from build123d import *

# Parameters (mm, degrees)
SKETCH1_W                                         = 133.096
SKETCH1_H                                         = 118.890132416
BOSS_EXTRUDE1_DEPTH                               = 10.16
SKETCH1_11_W                                      = 98.552
SKETCH1_11_H                                      = 57.404
SKETCH1_11_R                                      = 4.064
SKETCH1_11_W_2                                    = 18.542
SKETCH1_11_H_2                                    = 18.542
CUT_EXTRUDE1_DEPTH                                = 179.752998302
SKETCH1_12_R                                      = 13.75
SKETCH1_12_R_2                                    = 7.5
SKETCH1_12_R_3                                    = 4.064
CUT_EXTRUDE2_DEPTH                                = 1.7
CSK_FOR_M2_5_FLAT_HEAD_MACHINE_SCREW1_D           = 2.9
CSK_FOR_M2_5_FLAT_HEAD_MACHINE_SCREW1_DEPTH       = 5.08
CSK_FOR_M2_5_FLAT_HEAD_MACHINE_SCREW1_CSINK_D     = 5.5
CSK_FOR_M2_5_FLAT_HEAD_MACHINE_SCREW1_CSINK_ANGLE = 90
CSK_FOR_M2_5_FLAT_HEAD_MACHINE_SCREW1_TIP         = 0.871247898
SKETCH6_R                                         = 4.02
CUT_EXTRUDE3_DEPTH                                = 7.62


with BuildPart() as part:
    # Sketch1 → Boss-Extrude1 (new body)
    with BuildSketch(Plane.XY):
        with Locations((66.548, 59.445066208)):
            Rectangle(SKETCH1_W, SKETCH1_H)
    extrude(amount=-BOSS_EXTRUDE1_DEPTH)

    # Sketch1_11 → Cut-Extrude1 (cut, through all)
    with BuildSketch(Plane.XY):
        with Locations((78.74, 43.942)):
            Rectangle(SKETCH1_11_W, SKETCH1_11_H)
        with Locations((78.74, 98.4758)):
            Circle(SKETCH1_11_R)
        with Locations((16.289896793, 64.367970222)):
            Rectangle(SKETCH1_11_W_2, SKETCH1_11_H_2)
        with Locations((16.289896793, 42.362289183)):
            Rectangle(SKETCH1_11_W_2, SKETCH1_11_H_2)
        with BuildLine():
            Line((49.911, 74.803), (107.569, 74.803))
            ThreePointArc((107.569, 74.803), (110.744, 77.978), (107.569, 81.153))
            Line((107.569, 81.153), (49.911, 81.153))
            ThreePointArc((49.911, 81.153), (46.736, 77.978), (49.911, 74.803))
        make_face()
    extrude(amount=-CUT_EXTRUDE1_DEPTH, mode=Mode.SUBTRACT)

    # Sketch1_12 → Cut-Extrude2 (cut)
    # profile 1 of 3: a face of its own
    with BuildSketch(Plane.XY):
        with Locations((78.74, 98.4758)):
            Circle(SKETCH1_12_R)
        with Locations((78.74, 98.4758)):
            Circle(SKETCH1_12_R_2, mode=Mode.SUBTRACT)
    # profile 2 of 3: a face of its own
    with BuildSketch(Plane.XY):
        with Locations((78.74, 98.4758)):
            Circle(SKETCH1_12_R_2)
        with Locations((78.74, 98.4758)):
            Circle(SKETCH1_12_R_3, mode=Mode.SUBTRACT)
    # profile 3 of 3: a face of its own
    with BuildSketch(Plane.XY):
        with BuildLine():
            Line((49.911, 73.914), (107.569, 73.914))
            ThreePointArc((107.569, 73.914), (111.633, 77.978), (107.569, 82.042))
            Line((107.569, 82.042), (49.911, 82.042))
            ThreePointArc((49.911, 82.042), (45.847, 77.978), (49.911, 73.914))
        make_face()
        with BuildLine():
            ThreePointArc((107.569, 74.803), (110.744, 77.978), (107.569, 81.153))
            Line((107.569, 81.153), (49.911, 81.153))
            ThreePointArc((49.911, 81.153), (46.736, 77.978), (49.911, 74.803))
            Line((49.911, 74.803), (107.569, 74.803))
        make_face(mode=Mode.SUBTRACT)
    extrude(amount=-CUT_EXTRUDE2_DEPTH, mode=Mode.SUBTRACT)

    # CSK for M2.5 Flat Head Machine Screw1
    with Locations(Plane(origin=(0, 0, -10.16), x_dir=(-1, 0, 0), z_dir=(0, 0, -1))):
        with Locations((-109.250378399, 110.932782256), (-65.089376176, 110.932782256), (-6.474944958, 110.932782256), (-16.176873925, 29.217411756)):
            CounterSinkHole(CSK_FOR_M2_5_FLAT_HEAD_MACHINE_SCREW1_D / 2, CSK_FOR_M2_5_FLAT_HEAD_MACHINE_SCREW1_CSINK_D / 2, depth=CSK_FOR_M2_5_FLAT_HEAD_MACHINE_SCREW1_DEPTH, counter_sink_angle=CSK_FOR_M2_5_FLAT_HEAD_MACHINE_SCREW1_CSINK_ANGLE)
            with Locations((0, 0, -(CSK_FOR_M2_5_FLAT_HEAD_MACHINE_SCREW1_DEPTH + CSK_FOR_M2_5_FLAT_HEAD_MACHINE_SCREW1_TIP / 2))):  # 118° drill point
                Cone(0, CSK_FOR_M2_5_FLAT_HEAD_MACHINE_SCREW1_D / 2, CSK_FOR_M2_5_FLAT_HEAD_MACHINE_SCREW1_TIP, mode=Mode.SUBTRACT)

    # Sketch6 → Cut-Extrude3 (cut)
    # profile 1 of 2: a face of its own
    with BuildSketch(Plane(origin=(0, 0, -12.7), x_dir=(-1, 0, 0), z_dir=(0, 0, -1))):
        with BuildLine():
            Line((-130.556, 116.350132416), (-2.54, 116.350132416))
            Line((-2.54, 116.350132416), (-2.54, 111.755344215))
            ThreePointArc((-2.54, 111.755344215), (-10.494944958, 110.932782256), (-2.54, 110.110220296))
            Line((-2.54, 110.110220296), (-2.54, 75.184))
            Line((-2.54, 75.184), (-46.453892972, 75.184))
            ThreePointArc((-46.453892972, 75.184), (-45.899930629, 79.893554097), (-49.911, 82.423))
            Line((-49.911, 82.423), (-107.569, 82.423))
            ThreePointArc((-107.569, 82.423), (-111.580069371, 79.893554097), (-111.026107028, 75.184))
            Line((-111.026107028, 75.184), (-130.556, 75.184))
            Line((-130.556, 75.184), (-130.556, 116.350132416))
        make_face()
        with Locations((-109.250378399, 110.932782256)):
            Circle(SKETCH6_R, mode=Mode.SUBTRACT)
        with Locations((-65.089376176, 110.932782256)):
            Circle(SKETCH6_R, mode=Mode.SUBTRACT)
    # profile 2 of 2: a face of its own
    with BuildSketch(Plane(origin=(0, 0, -12.7), x_dir=(-1, 0, 0), z_dir=(0, 0, -1))):
        with BuildLine():
            Line((-26.924, 30.551289183), (-26.924, 2.54))
            Line((-26.924, 2.54), (-2.54, 2.54))
            Line((-2.54, 2.54), (-2.54, 30.551289183))
            Line((-2.54, 30.551289183), (-12.384622481, 30.551289183))
            ThreePointArc((-12.384622481, 30.551289183), (-16.176873925, 25.197411756), (-19.969125368, 30.551289183))
            Line((-19.969125368, 30.551289183), (-26.924, 30.551289183))
        make_face()
    extrude(amount=-CUT_EXTRUDE3_DEPTH, mode=Mode.SUBTRACT)


solid = part.part
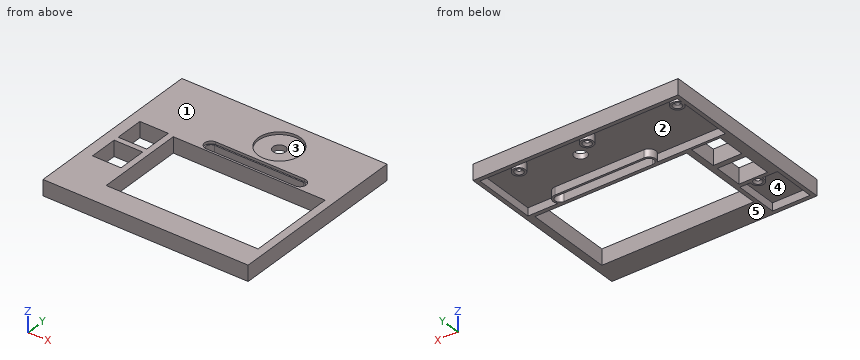
Verification items for the finished model (mm, model axes). Face numbers are marked on the shaded views. A direction names the side the tool comes from. Give positions to 0.01 mm unless a question says otherwise; leave off trailing zeros. Loops run counter-clockwise (first coordinate to the right, second up) from the corner with the lowest first, then second, coordinate; pieces in that order, holes last.
1) Sectioned sample at C-C, the plane x = 54. Enter the section's corners in (y, z), then the cut area to 3 significant figures.
2) Sectioned sample at B-B, the plane y = 42. Enter the section's corners in (x, z), then the cut area to 3 significant figures.
3) Sectioned sample at D-D, the plane x = 78.74. Enter the section's corners in (y, z).
4) Depth check by flat-ended pin: pin 1 Ø4 at (x, y) = (16, 57.5) entering from -Z; pin 2 Ø4 at (x, y) = (109.25, 110.93) entering from -Z. Enter the tip coordinate at first touch or a pass-through.
5) Thickness scan on line 1 along X through (y, z) = (66, -5.5); line 2 along Y through (x, z) = (107, -1); line 3 along Y through (x, z) = (10.5, -1.25). Record the ranges inside material, lowest first.
6) Sectioned sample at A-A, the plane x = 122.5. Enter the section's corners in (y, z).
7) Set-up check for the marked faces 1, 2 and 3: record each of +Z, -Z, +X, -X, +Y, -Y from which the full face is reachable in a straight line by a thin tool's end or side.
8) Draft check along X on the marked faces 4 and 5. Enter one of: pulls with the +X half, pulls with the -X half, needs draft (parallel to the pull), parting line crosses it, or undercut.
Answers:
1. outline: (0, -10.16) - (15.24, -10.16) - (15.24, 0) - (0, 0) - close; (72.64, -10.16) - (74.8, -10.16) - (74.8, -1.7) - (73.91, -1.7) - (73.91, 0) - (72.64, 0) - close; (81.15, -10.16) - (82.42, -10.16) - (82.42, -5.08) - (116.35, -5.08) - (116.35, -10.16) - (118.89, -10.16) - (118.89, 0) - (82.04, 0) - (82.04, -1.7) - (81.15, -1.7) - close
1. area: 385 mm2
2. outline: (0, -10.16) - (7.02, -10.16) - (7.02, 0) - (0, 0) - close; (25.56, -10.16) - (29.46, -10.16) - (29.46, 0) - (25.56, 0) - close; (128.02, -10.16) - (133.1, -10.16) - (133.1, 0) - (128.02, 0) - close
2. area: 163 mm2
3. outline: (0, -10.16) - (15.24, -10.16) - (15.24, 0) - (0, 0) - close; (72.64, -10.16) - (74.8, -10.16) - (74.8, -1.7) - (73.91, -1.7) - (73.91, 0) - (72.64, 0) - close; (81.15, -10.16) - (82.42, -10.16) - (82.42, -5.08) - (94.41, -5.08) - (94.41, -1.7) - (84.73, -1.7) - (84.73, 0) - (82.04, 0) - (82.04, -1.7) - (81.15, -1.7) - close; (102.54, -5.08) - (116.35, -5.08) - (116.35, -10.16) - (118.89, -10.16) - (118.89, 0) - (112.23, 0) - (112.23, -1.7) - (102.54, -1.7) - close
4. pin 1: passes through
4. pin 2: stops at z = -9.41
5. line 1: x = 0 to 7.02, 25.56 to 29.46, 128.02 to 133.1
5. line 2: y = 0 to 15.24, 72.64 to 73.91, 82.04 to 118.89
5. line 3: y = 0 to 33.09, 51.63 to 55.1, 73.64 to 118.89
6. outline: (0, -10.16) - (15.24, -10.16) - (15.24, 0) - (0, 0) - close; (72.64, -10.16) - (75.18, -10.16) - (75.18, -5.08) - (116.35, -5.08) - (116.35, -10.16) - (118.89, -10.16) - (118.89, 0) - (72.64, 0) - close
7. face 1: +Z, +X, -X, +Y, -Y
7. face 2: -Z
7. face 3: +Z
8. face 4: undercut
8. face 5: needs draft
